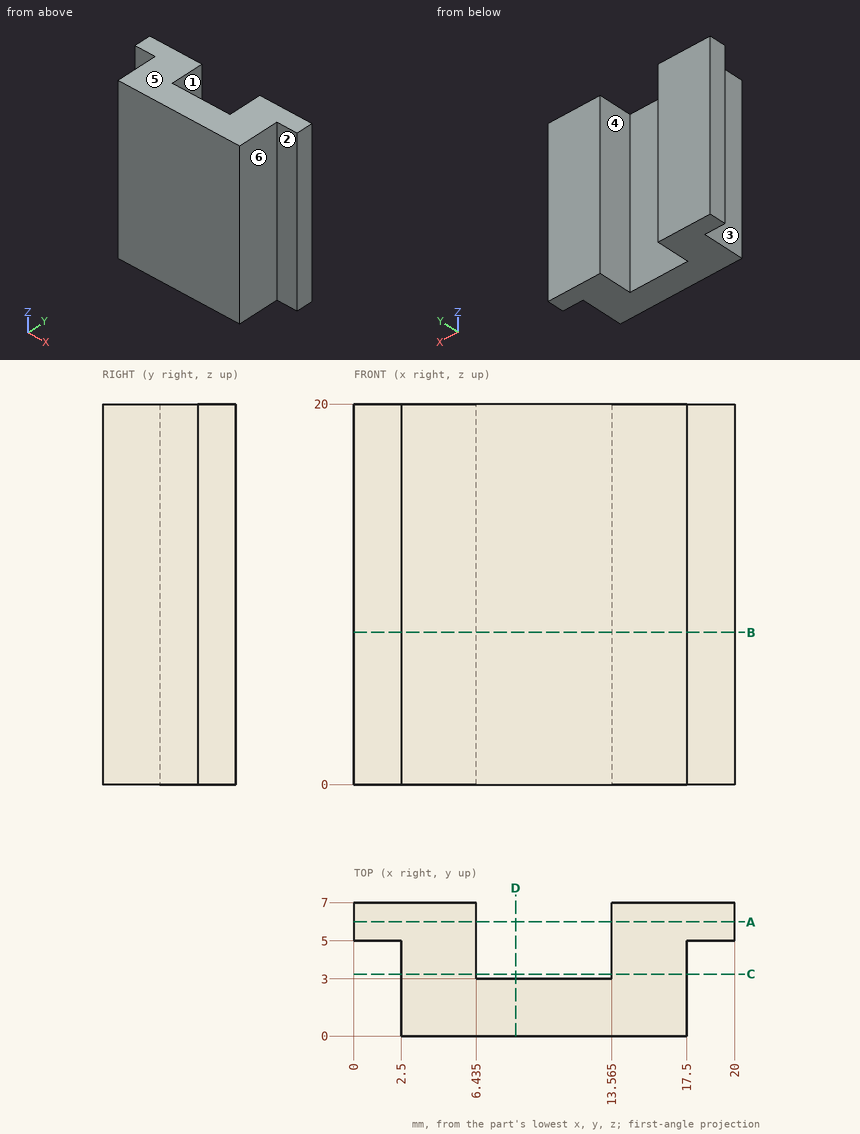
Can you work these out from the drawing? Everything is in mm from the part's minimum corner. A direction names the side the tool comes from. Round coordinates to 2 decimals unless told otherwise and drop trailing zeros. Loops run counter-clockwise (first coordinate to the right, second up) from the corner with the lowest first, then second, coordinate; pieces in that order, holes last. Notation, with made-up numbers: (31.5, 68) -> (49.5, 68) arc R19 ccw to (49.5, 82) -> close; hole circle Ø6 at (-20, 49). An arc over 180 degrees is marked (long way). Use CSV: the item, a comma, the result in double quotes.
(1) If we mould it in two halves opening along X, with no side actions, what happens to the marked faces 4, 5 and 6? For each: +X half, -X half, draft (parallel to the pull), parting line (faces both ways), or undercut.
Return value:
face 4,"undercut"
face 5,"draft"
face 6,"+X half"
(2) Suppose I cut it at A-A on y = 6. Write out the boundary of the cut face in (x, z) (3 decimals), plus the area to 3 significant figures.
Return value:
outline,"(0, 0) -> (6.435, 0) -> (6.435, 20) -> (0, 20) -> close; (13.565, 0) -> (20, 0) -> (20, 20) -> (13.565, 20) -> close"
area,"257 mm²"
(3) Suppose I cut it at C-C on y = 3.25. Write out the boundary of the cut face in (x, z) (3 decimals).
Return value:
outline,"(2.5, 0) -> (6.435, 0) -> (6.435, 20) -> (2.5, 20) -> close; (13.565, 0) -> (17.5, 0) -> (17.5, 20) -> (13.565, 20) -> close"
(4) For the marked faces 1, 2 and 3, which set-ups out of +Z, -Z, +X, -X, +Y, -Y let a thin tool reach every point of the face, with its end or its side?
Return value:
face 1,"+Z, -Z, +Y"
face 2,"+Z, -Z, +X, -Y"
face 3,"+Z, -Z, -X, -Y"
(5) Will these pins go through, and if not, where does the flat tip stop? pin 1 Ø1.5 at (y, z) = (2.5, 9.5) entering from +X; pin 2 Ø1.5 at (y, z) = (2, 13) entering from -X; pin 3 Ø1.2 at (x, z) = (1.5, 6) entering from -Y.
Return value:
pin 1,"stops at x = 17.5"
pin 2,"stops at x = 2.5"
pin 3,"stops at y = 5"
(6) Suppose I cut it at D-D on x = 8.5. Write out the boundary of the cut face in (y, z), plus the area to 3 significant figures.
Return value:
outline,"(0, 0) -> (3, 0) -> (3, 20) -> (0, 20) -> close"
area,"60.0 mm²"
(7) If I drill on probe 1 along X at (y, z) = (3.25, 18.75) (3 decimals); probe 2 along X at (y, z) = (5.25, 16) (3 decimals); probe 3 along Y at (x, z) = (9.75, 12.75), over which ranges is the centre line in solid material (lowest first)? Write a range as [from, to].
Return value:
probe 1,"x = [2.5, 6.435], [13.565, 17.5]"
probe 2,"x = [0, 6.435], [13.565, 20]"
probe 3,"y = [0, 3]"
(8) Suppose I cut it at B-B on z = 8. Write out the boundary of the cut face in (x, y) (3 decimals).
Return value:
outline,"(0, 5) -> (2.5, 5) -> (2.5, 0) -> (17.5, 0) -> (17.5, 5) -> (20, 5) -> (20, 7) -> (13.565, 7) -> (13.565, 3) -> (6.435, 3) -> (6.435, 7) -> (0, 7) -> close"
